The drawing under review shows one solid part. Ordinate dimensions are in mm from its lowest x, y, z. Give positions to 0.01 mm unless a question says otherwise; leave off trailing zeros. Loops run counter-clockwise (first coordinate to the right, second up) from the corner with the lowest first, then second, coordinate; pieces in that order, holes last. Notation, with made-up numbers: M 1.5,-32.5 L 28.5,-32.5 A28 cw 28.5,-13.5 Z; hole C 3.25,-27.75 d9. An arc over 180 degrees is marked long. One line per item, written item: value. Start each with the question number.
Q1. We need section B-B on x = 119. Write out the cut boundary in (y, z), plus the area to 3 significant figures.
Q2. We need section A-A on y = 49.5. Write out the cut boundary in (x, z), plus the area to 3 significant figures.
Q3. To check wall thickness, follow line 1 along Y through (x, z) = (20, 7.15); line 2 along Y through (x, z) = (137.5, 8.25); line 3 along X through (y, z) = (33.5, 6) (1 decimal). State the ranges of each line that lie inside material, in increasing order. Write a range as from..to.
Q4. For pin 1 (8 mm diameter, centred on y = 10.5, z = 5, fed in from -X) (1 decimal); pin 2 (3 mm diameter, centred on y = 16, z = 3, fed in from +X) (1 decimal); pin 3 (1 mm diameter, centred on x = 120, y = 21.5, fed in from -Z), all flat-tipped, find the tip position at first contact; note any pin that passes through.
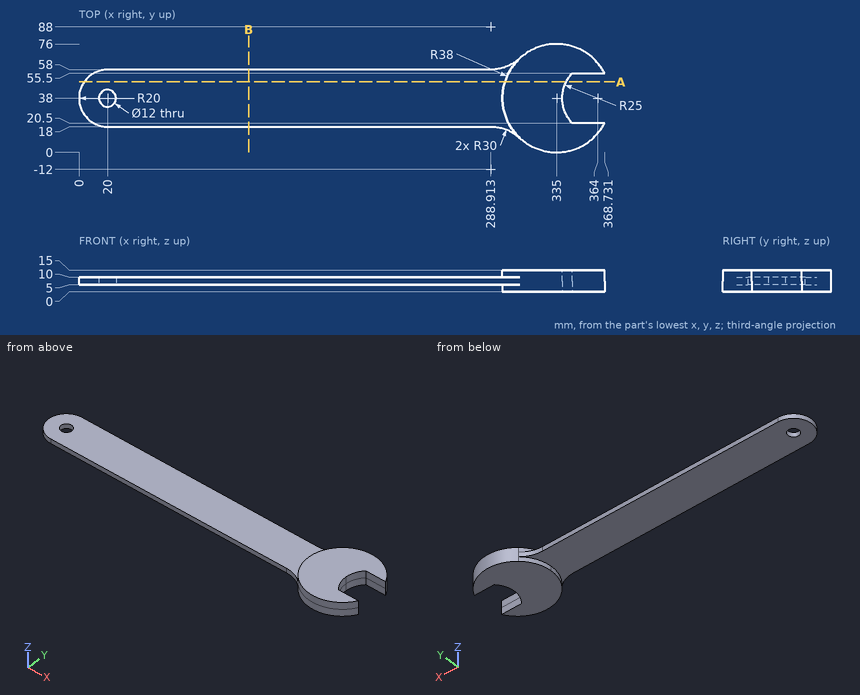
Solved:
1. outline: M 18,5 L 58,5 L 58,10 L 18,10 Z
1. area: 200 mm2
2. outline: M 3.64,5 L 298.78,5 L 298.78,0 L 341.8,0 L 341.8,15 L 298.78,15 L 298.78,10 L 3.64,10 Z
2. area: 2,120 mm2
3. line 1: 18..32, 44..58
3. line 2: 18..58
3. line 3: 0.5..16, 24..339.4
4. pin 1: x = 303
4. pin 2: x = 367
4. pin 3: z = 5
